Geometry check sheet. Reference: the model listing, model coordinates, mm. A direction names the side the tool comes from. Coordinates: 2 decimals unless noted, no trailing zeros. Order: outer loops, then holes, each group sorted by start corner. A loop starts at its lowest first (then second) coordinate and runs counter-clockwise, first axis right, second up. Notation, with made-up numbers: (63, -39.5) - (105, -39.5) arc R34 cw to (105, -4.5) - close; hole circle Ø3 at (-6.5, 77.5). An arc over 180 degrees is marked (long way). Return JSON: item names as keys, results as strings. Group by question number.
Item 1: Section check C-C on z = -64.5. Enter the section's corners in (x, y).
Item 2: Section check A-A on y = -86. Enter the section's corners in (x, z), then the cut area to 3 significant figures.
Item 3: Gauge pin test, flat ends, axial feed: pin 1 (6 mm diameter, centred on x = 708.5, z = -216, fed in from -Y); pin 2 (3 mm diameter, centred on y = -209.5, z = -170, fed in from -X); pin 3 (2 mm diameter, centred on x = 587.5, y = -173.5, fed in from +Z); pin 4 (4 mm diameter, centred on y = -164, z = -272, fed in from -X). Record the tip position at first contact, or that the pin passes through.
Item 4: Section check D-D on x = 607.5. Give the number of separate pieces and of enclosed holes in the cut face, then the cut area to 3 significant figures.
Item 5: Section check B-B on y = -561. Enter the section's corners in (x, z), then the cut area to 3 significant figures.
Item 6: Tool access check on faces 4 (the flat face through (76.2, -552, -150)), 5 (the flat face through (38.1, -552, -152)), 6 (the flat face through (858, -266.7, -155)), 7 (the flat face through (57, -177.8, -37)). Record the directions out of +Z, -Z, +X, -X, +Y, -Y that give a thin tool (end or side, any length) a straight path to the whole face; none if there is none.
Item 7: Scan lines: probe 1 along Y at (x, z) = (635.5, -139.5); probe 2 along Z at (x, y) = (854, -505.5); probe 3 along Y at (x, z) = (65.5, -235). Record each from-to range of solid material in increasing order.
Item 8: Draft check along Z on faces 1 (the flat face through (455, 24, 0)), 2 (the flat face through (452, -508, -212)), 3 (the flat face through (57, -508, -135)). Enter one of: pulls with the +Z half, pulls with the -Z half, needs draft (parallel to the pull), parting line crosses it, or undercut.
from build123d import *

# Parameters (mm, degrees)
SKETCH1_W            = 914.4
SKETCH1_H            = 304.8
BOSS_EXTRUDE3_DEPTH  = 38.1
SKETCH5_W            = 38.1
SKETCH5_H            = 88.9
BOSS_EXTRUDE4_DEPTH  = 660.4
SKETCH7_W            = 304.8
SKETCH7_H            = 88.9
BOSS_EXTRUDE5_DEPTH  = 38.1
SKETCH6_W            = 304.8
SKETCH6_H            = 88.9
BOSS_EXTRUDE6_DEPTH  = 38.1
SKETCH9_W            = 304.8
SKETCH9_H            = 88.9
BOSS_EXTRUDE7_DEPTH  = 38.1
SKETCH8_W            = 304.8
SKETCH8_H            = 88.9
BOSS_EXTRUDE8_DEPTH  = 38.1
SKETCH10_W           = 838.2
SKETCH10_H           = 19.05
SKETCH10_W_2         = 838.173774045
SKETCH10_W_3         = 838.158204612
SKETCH10_W_4         = 838.175626617
SKETCH10_W_5         = 838.17389523
BOSS_EXTRUDE9_DEPTH  = 19.05
SKETCH11_W           = 838.2
SKETCH11_H           = 19.05
SKETCH11_H_2         = 19.304
BOSS_EXTRUDE10_DEPTH = 19.05


with BuildPart() as part:
    # Sketch1 → Boss-Extrude3 (new body)
    with BuildSketch(Plane(origin=(0, 0, 0), x_dir=(1, 0, 0), z_dir=(0, 1, 0))):
        with Locations((457.2, 152.4)):
            Rectangle(SKETCH1_W, SKETCH1_H)
    extrude(amount=BOSS_EXTRUDE3_DEPTH)

    # Sketch5 → Boss-Extrude4 (add)
    with BuildSketch(Plane.XZ):
        with Locations((19.05, -44.45)):
            Rectangle(SKETCH5_W, SKETCH5_H)
        with Locations((19.05, -260.35)):
            Rectangle(SKETCH5_W, SKETCH5_H)
        with Locations((895.35, -44.45)):
            Rectangle(SKETCH5_W, SKETCH5_H)
        with Locations((895.35, -260.35)):
            Rectangle(SKETCH5_W, SKETCH5_H)
    extrude(amount=BOSS_EXTRUDE4_DEPTH)

    # Sketch7 → Boss-Extrude5 (add)
    with BuildSketch(Plane(origin=(38.1, 0, 0), x_dir=(0, 0, -1), z_dir=(1, 0, 0))):
        with Locations((152.4, -222.25)):
            Rectangle(SKETCH7_W, SKETCH7_H)
    extrude(amount=BOSS_EXTRUDE5_DEPTH)

    # Sketch6 → Boss-Extrude6 (add)
    with BuildSketch(Plane.ZY.offset(-876.3)):
        with Locations((-152.4, -222.25)):
            Rectangle(SKETCH6_W, SKETCH6_H)
    extrude(amount=BOSS_EXTRUDE6_DEPTH)

    # Sketch9 → Boss-Extrude7 (add)
    with BuildSketch(Plane.ZY.offset(-876.3)):
        with Locations((-152.4, -552.45)):
            Rectangle(SKETCH9_W, SKETCH9_H)
    extrude(amount=BOSS_EXTRUDE7_DEPTH)

    # Sketch8 → Boss-Extrude8 (add)
    with BuildSketch(Plane(origin=(38.1, 0, 0), x_dir=(0, 0, -1), z_dir=(1, 0, 0))):
        with Locations((152.4, -552.45)):
            Rectangle(SKETCH8_W, SKETCH8_H)
    extrude(amount=BOSS_EXTRUDE8_DEPTH)

    # Sketch10 → Boss-Extrude9 (add)
    with BuildSketch(Plane(origin=(0, -508, 0), x_dir=(1, 0, 0), z_dir=(0, 1, 0))):
        with Locations((457.2, 269.875)):
            Rectangle(SKETCH10_W, SKETCH10_H)
        with Locations((457.180463347, 211.855946701)):
            Rectangle(SKETCH10_W_2, SKETCH10_H)
        with Locations((457.188248064, 144.838690295)):
            Rectangle(SKETCH10_W_3, SKETCH10_H)
        with Locations((457.155340061, 83.805117496)):
            Rectangle(SKETCH10_W_4, SKETCH10_H)
        with Locations((457.213052385, 25.16501814)):
            Rectangle(SKETCH10_W_5, SKETCH10_H)
    extrude(amount=BOSS_EXTRUDE9_DEPTH)

    # Sketch11 → Boss-Extrude10 (add)
    with BuildSketch(Plane(origin=(0, -177.8, 0), x_dir=(1, 0, 0), z_dir=(0, 1, 0))):
        with Locations((457.2, 269.875)):
            Rectangle(SKETCH11_W, SKETCH11_H)
        with Locations((457.2, 212.725)):
            Rectangle(SKETCH11_W, SKETCH11_H)
        with Locations((457.2, 144.78)):
            Rectangle(SKETCH11_W, SKETCH11_H_2)
        with Locations((457.2, 83.841878729)):
            Rectangle(SKETCH11_W, SKETCH11_H_2)
        with Locations((457.283867399, 24.910423168)):
            Rectangle(SKETCH11_W, SKETCH11_H_2)
    extrude(amount=BOSS_EXTRUDE10_DEPTH)


solid = part.part
Computed:
{
 "1": {"outline": "(0, -660.4) - (38.1, -660.4) - (38.1, -596.9) - (76.2, -596.9) - (76.2, -508) - (38.1, -508) - (38.1, -266.7) - (76.2, -266.7) - (76.2, -177.8) - (38.1, -177.8) - (38.1, 0) - (876.3, 0) - (876.3, -177.8) - (838.2, -177.8) - (838.2, -266.7) - (876.3, -266.7) - (876.3, -508) - (838.2, -508) - (838.2, -596.9) - (876.3, -596.9) - (876.3, -660.4) - (914.4, -660.4) - (914.4, 38.1) - (0, 38.1) - close"},
 "2": {"outline": "(0, -304.8) - (38.1, -304.8) - (38.1, -215.9) - (0, -215.9) - close; (0, -88.9) - (38.1, -88.9) - (38.1, 0) - (0, 0) - close; (876.3, -304.8) - (914.4, -304.8) - (914.4, -215.9) - (876.3, -215.9) - close; (876.3, -88.9) - (914.4, -88.9) - (914.4, 0) - (876.3, 0) - close", "area": "13,500 mm²"},
 "3": {"pin 1": "stops at y = -508", "pin 2": "stops at x = 38.1", "pin 3": "stops at z = -15.26", "pin 4": "stops at x = 0"},
 "4": {"separate pieces": "11", "enclosed holes": "0", "area": "15,300 mm²"},
 "5": {"outline": "(0, -304.8) - (76.2, -304.8) - (76.2, 0) - (0, 0) - (0, -88.9) - (38.1, -88.9) - (38.1, -215.9) - (0, -215.9) - close; (838.2, -304.8) - (914.4, -304.8) - (914.4, -215.9) - (876.3, -215.9) - (876.3, -88.9) - (914.4, -88.9) - (914.4, 0) - (838.2, 0) - close", "area": "36,800 mm²"},
 "6": {"face 4": "+Z, -Z, -Y", "face 5": "-X, -Y", "face 6": "+Z, -Z", "face 7": "none"},
 "7": {"probe 1": "y = -508 to -488.95, -177.8 to -158.75, 0 to 38.1", "probe 2": "z = -279.4 to -260.35, -221.38 to -202.33, -154.36 to -135.31, -93.33 to -74.28, -34.69 to -15.64", "probe 3": "y = -596.9 to -508, -266.7 to -177.8, 0 to 38.1"},
 "8": {"face 1": "pulls with the +Z half", "face 2": "needs draft", "face 3": "undercut"}
}
